CAD build for the part. Positions are in the model's coordinates, mm. Face numbers are marked on the shaded views. A direction names the side the tool comes from. Round coordinates to 2 decimals unless told otherwise and drop trailing zeros. Loops run counter-clockwise (first coordinate to the right, second up) from the corner with the lowest first, then second, coordinate; pieces in that order, holes last. Notation, with made-up numbers: M 50,3 L 93,3 A10 ccw 93,19 Z; hole C 62,16.5 d2. An arc over 180 degrees is marked long. Use one line per item in the form item = value.
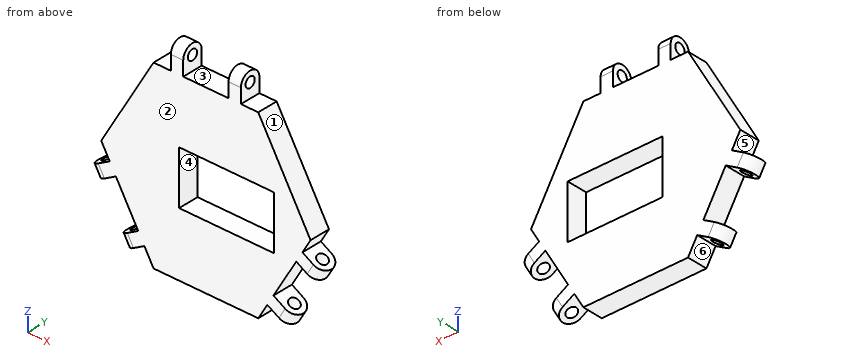
from build123d import *

# Parameters (mm, degrees)
BOSS_EXTRUDE1_DEPTH     = 5
BOSS_EXTRUDE2_START     = 5.5
SKETCH2_R               = 1.25
BOSS_EXTRUDE2_DEPTH     = 3
CIRPATTERN1_START       = -8.29907709
CIRPATTERN1_OUTLINE_R   = 1.25
CIRPATTERN1_DEPTH       = 3
CIRPATTERN1_START_2     = 5.754432
CIRPATTERN1_2_OUTLINE_R = 1.25
CIRPATTERN1_2_DEPTH     = 3
CIRPATTERN1_START_3     = -8.588604314
CIRPATTERN1_3_OUTLINE_R = 1.25
CIRPATTERN1_3_DEPTH     = 3
CIRPATTERN1_START_4     = 5.245568
CIRPATTERN1_4_OUTLINE_R = 1.25
CIRPATTERN1_4_DEPTH     = 3
CUT_EXTRUDE1_REACH      = 42.122
SKETCH3_W               = 23
SKETCH3_H               = 13


# Read off the part's stored shape, not the designer's step: CirPattern1
with BuildPart() as part:
    # Sketch1 → Boss-Extrude1 (new body)
    with BuildSketch(Plane(origin=(0, 0, 0), x_dir=(1, 0, 0), z_dir=(0, 1, 0))):
        Polygon((25.403411844, 0), (12.701705922, 22), (-12.701705922, 22), (-25.403411844, 0), (-12.701705922, -22), (12.701705922, -22), align=None)
    extrude(amount=BOSS_EXTRUDE1_DEPTH)

    # Sketch2 → Boss-Extrude2 (add)
    with BuildSketch(Plane(origin=(0, 0, 0), x_dir=(0, 0, -1), z_dir=(1, 0, 0)).offset(BOSS_EXTRUDE2_START)):
        with BuildLine():
            Line((-22, 5), (-25.5, 5))
            ThreePointArc((-25.5, 5), (-28, 2.5), (-25.5, 0))
            Line((-25.5, 0), (-22, 0))
            Line((-22, 0), (-22, 5))
        make_face()
        with Locations((-25.5, 2.5)):
            Circle(SKETCH2_R, mode=Mode.SUBTRACT)
    boss_extrude2 = extrude(amount=BOSS_EXTRUDE2_DEPTH)

    # Mirror1: Boss-Extrude2 across plane
    add(boss_extrude2.mirror(Plane(origin=(0, 0, 0), x_dir=(0, 0, 1), z_dir=(1, 0, 0))))

    # CirPattern1 outline → CirPattern1 (add)
    with BuildSketch(Plane(origin=(0, 0, 0), x_dir=(0.8660254037844362, 0, -0.5000000000000042), z_dir=(0.5000000000000042, 0, 0.8660254037844363)).offset(CIRPATTERN1_START)):
        with BuildLine():
            Line((25.281685655, 5), (22, 5))
            Line((22, 5), (22, 0))
            Line((22, 0), (25.281685655, 0))
            ThreePointArc((25.281685655, 0), (27.781685655, 2.5), (25.281685655, 5))
        make_face()
        with Locations((25.281685655, 2.5)):
            Circle(CIRPATTERN1_OUTLINE_R, mode=Mode.SUBTRACT)
    extrude(amount=CIRPATTERN1_DEPTH)

    # CirPattern1 2 outline → CirPattern1 2 (add)
    with BuildSketch(Plane(origin=(0, 0, 0), x_dir=(0.8660254037844362, 0, -0.5000000000000042), z_dir=(0.5000000000000042, 0, 0.8660254037844363)).offset(CIRPATTERN1_START_2)):
        with BuildLine():
            ThreePointArc((25.059310849, 0), (27.559310849, 2.5), (25.059310849, 5))
            Line((25.059310849, 5), (22, 5))
            Line((22, 5), (22, 0))
            Line((22, 0), (25.059310849, 0))
        make_face()
        with Locations((25.059310849, 2.5)):
            Circle(CIRPATTERN1_2_OUTLINE_R, mode=Mode.SUBTRACT)
    extrude(amount=CIRPATTERN1_2_DEPTH)

    # CirPattern1 3 outline → CirPattern1 3 (add)
    with BuildSketch(Plane(origin=(0, 0, 0), x_dir=(0.8660254037844431, 0, 0.4999999999999921), z_dir=(0.4999999999999921, 0, -0.8660254037844433)).offset(CIRPATTERN1_START_3)):
        with BuildLine():
            Line((-25.216838483, -5), (-22, -5))
            Line((-22, -5), (-22, 0))
            Line((-22, 0), (-25.216838483, 0))
            ThreePointArc((-25.216838483, 0), (-27.716838483, -2.5), (-25.216838483, -5))
        make_face()
        with Locations((-25.216838483, -2.5)):
            Circle(CIRPATTERN1_3_OUTLINE_R, mode=Mode.SUBTRACT)
    extrude(amount=CIRPATTERN1_3_DEPTH)

    # CirPattern1 4 outline → CirPattern1 4 (add)
    with BuildSketch(Plane(origin=(0, 0, 0), x_dir=(0.8660254037844431, 0, 0.4999999999999921), z_dir=(0.4999999999999921, 0, -0.8660254037844433)).offset(CIRPATTERN1_START_4)):
        with BuildLine():
            ThreePointArc((-25.059310849, 0), (-27.559310849, -2.5), (-25.059310849, -5))
            Line((-25.059310849, -5), (-22, -5))
            Line((-22, -5), (-22, 0))
            Line((-22, 0), (-25.059310849, 0))
        make_face()
        with Locations((-25.059310849, -2.5)):
            Circle(CIRPATTERN1_4_OUTLINE_R, mode=Mode.SUBTRACT)
    extrude(amount=CIRPATTERN1_4_DEPTH)

    # Sketch3 → Cut-Extrude1 (cut, up to next)
    with BuildSketch(Plane(origin=(0, 5, 0), x_dir=(1, 0, 0), z_dir=(0, 1, 0)), mode=Mode.PRIVATE) as cut_extrude1_sk1:
        with Locations((5, 0)):
            Rectangle(SKETCH3_W, SKETCH3_H)
    cut_extrude1_tool1 = extrude(cut_extrude1_sk1.sketch, amount=-CUT_EXTRUDE1_REACH, mode=Mode.PRIVATE) & part.part
    add(cut_extrude1_tool1.solids().sort_by_distance((5, 5, 0))[0], mode=Mode.SUBTRACT)


solid = part.part
1. Cut at B-B on z = 3. Write the cut outline in (x, y), and give its area (3 significant figures).
Completed:
outline = M -23.67,0 L -6.5,0 L -6.5,5 L -23.67,5 Z; M 16.5,0 L 23.67,0 L 23.67,5 L 16.5,5 Z
area = 122 mm2
2. Pull direction X, two halves, no side cores. Call the marked faces 1, 2 and 3: +X half, -X half, draft (parallel to the pull), parting line (faces both ways), or undercut.
Completed:
face_1 = +X half
face_2 = draft
face_3 = undercut
3. Cut at A-A on x = 0. Write the cut outline in (y, z), and give its area (3 significant figures).
Completed:
outline = M 0,-22 L 5,-22 L 5,-6.5 L 0,-6.5 Z; M 0,6.5 L 5,6.5 L 5,22 L 0,22 Z
area = 155 mm2
4. Tool access for the marked faces 4, 5 and 6: list every direction of +Z, -Z, +X, -X, +Y, -Y with a clear straight run to the whole face (end or side of a thin tool).
Completed:
face_4 = +Y, -Y
face_5 = -X, +Y, -Y
face_6 = -Z, +Y, -Y
5. Cut at C-C on y = 2.5. State how many separate pieces and enclosed holes the cut face has, and give its area (3 significant figures).
Completed:
separate_pieces = 7
enclosed_holes = 1
area = 1,440 mm2
6. Drop flat-ended pins along their axis: P1, Ø1.5, axis at x = 1, y = 3.5, coming from the +Z side; P2, Ø2.5, axis at y = 2.5, z = 24.5, coming from the +X side; P3, Ø2.5, axis at y = 1.5, z = 24.5, coming from the -X side; P4, Ø2, axis at y = 2.5, z = 25.5, coming from the -X side. Give the stop position or say it passes through.
Completed:
P1 = 22
P2 = 8.5
P3 = -8.5
P4 = through
7. Cut at D-D on z = -10.5. Write the cut outline in (x, y).
Completed:
outline = M -19.34,0 L 19.34,0 L 19.34,5 L -19.34,5 Z
8. Probe line 1 along Z through (x, y) = (4, 1); line 2 along Y through (x, z) = (7.55, 25.5); line 3 along X through (y, z) = (1.9, -19). List the from-to ranges inside material, lowest first. Write a range as from..to.
Completed:
line_1 = -22..-6.5, 6.5..22
line_2 = 0..1.25, 3.75..5
line_3 = -20.77..-19.23, -16.7..-16.42, -14.43..14.43, 16.31..16.96, 19.49..21.03
